For this review, take the finished solid that the model builds, in its own axes (mm). Give positions to 0.01 mm unless a question says otherwise; leave off trailing zeros. Loops run counter-clockwise (first coordinate to the right, second up) from the corner with the lowest first, then second, coordinate; pieces in that order, holes last. Notation, with made-up numbers: (3.25, 18.5) - (60.25, 18.5) arc R23 cw to (60.25, 31.5) - close; hole circle Ø5 at (12.5, 32.25). An arc over 180 degrees is marked (long way). Answer in a Markdown table with one row per item.
Autodesk Inventor part; units mm, degrees
ref_plane "YZ Plane" through (0, 0, 0) normal (1, 0, 0) x (0, 1, 0)
ref_plane "XZ Plane" through (0, 0, 0) normal (0, 1, 0) x (-1, 0, 0)
ref_plane "XY Plane" through (0, 0, 0) normal (0, 0, 1) x (1, 0, 0)
sketch "Sketch1" plane through (0, 0, 0) normal (0, 0, 1) x (1, 0, 0)
  circle A0 centre (-0.1245, -8) radius 2.5
  circle A1 centre (-0.018, 28) radius 2.5
  line L0 (-20, 40) -> (-20, -45)
  line L1 (-20, -45) -> (20, -45)
  line L2 (20, -45) -> (20, 40)
  circle A2 centre (-0.1245, -8) radius 2.5
  circle A3 centre (-0.018, 28) radius 2.5
  line L3 (20, -45) -> (-20, -45)
  line L4 (-20, -45) -> (-20, 75)
  line L5 (-20, 75) -> (20, 75)
  line L6 (20, 75) -> (20, -45)
  circle A4 centre (0, 10) radius 4
  point P0 (0, 0)
  point P1 (20, 40)
  dimension "d0" = 120
  dimension "d1" = 8
extrude "Extrusion1" add sketch "Sketch1" along normal blind 6
properties part number "gard1" material "PMMA Plastic"
1. Wall thickness on line 1 (Y direction, x = 0, z = 1.3); line 2 (Y direction, x = -3.5, z = 4.95): over which ranges is each line inside the solid? List them lowest first. Write a range as [from, to].
Values:
| item | result |
|---|---|
| line 1 | y = [-45, -10.5], [-5.5, 6], [14, 25.5], [30.5, 75] |
| line 2 | y = [-45, 8.06], [11.94, 75] |
2. We need section A-A, the plane y = 10. Give the boundary of the cut face in (x, z), and give its area (3 significant figures).
Values:
| item | result |
|---|---|
| outline | (-20, 0) - (-4, 0) - (-4, 6) - (-20, 6) - close; (4, 0) - (20, 0) - (20, 6) - (4, 6) - close |
| area | 192 mm^2 |
3. We need section D-D, the plane y = 28. Give the boundary of the cut face in (x, z), and give its area (3 significant figures).
Values:
| item | result |
|---|---|
| outline | (-20, 0) - (-2.52, 0) - (-2.52, 6) - (-20, 6) - close; (2.48, 0) - (20, 0) - (20, 6) - (2.48, 6) - close |
| area | 210 mm^2 |
4. We need section C-C, the plane x = 0. Give the boundary of the cut face in (y, z), and give its area (3 significant figures).
Values:
| item | result |
|---|---|
| outline | (-45, 0) - (-10.5, 0) - (-10.5, 6) - (-45, 6) - close; (-5.5, 0) - (6, 0) - (6, 6) - (-5.5, 6) - close; (14, 0) - (25.5, 0) - (25.5, 6) - (14, 6) - close; (30.5, 0) - (75, 0) - (75, 6) - (30.5, 6) - close |
| area | 612 mm^2 |
5. We need section B-B, the plane z = 3.85. Give the boundary of the cut face in (x, y), and give its area (3 significant figures).
Values:
| item | result |
|---|---|
| outline | (-20, -45) - (20, -45) - (20, 75) - (-20, 75) - close; hole circle Ø8 at (0, 10); hole circle Ø5 at (-0.12, -8); hole circle Ø5 at (-0.02, 28) |
| area | 4,710 mm^2 |
6. Mouldability with a two-part tool opening along X and no side actions: class faces 1 (the face through (-0.867, 13.905, 2.958)), 2 (the face through (0, 16, 6)), 3 (the face through (20, 14, 3)) as released by +X, released by -X, zero draft, split by the parting line, or undercut.
Values:
| item | result |
|---|---|
| face 1 | undercut |
| face 2 | zero draft |
| face 3 | released by +X |
